from build123d import *

# Parameters (mm, degrees)
EXTRUDE_1_DEPTH = 2000


with BuildPart() as part:
    # Эскиз1 → Вытянуть-Тонкостенный1 (new body)
    with BuildSketch(Plane(origin=(0, 0, 0), x_dir=(0, 0, -1), z_dir=(1, 0, 0))):
        Polygon((-18, -0.2), (0.110849528, -0.2), (5.110849528, 7.8), (57.389150472, 7.8), (62.389150472, -0.2), (115.110849528, -0.2), (120.110849528, 7.8), (172.389150472, 7.8), (177.389150472, -0.2), (230.110849528, -0.2), (235.110849528, 7.8), (287.389150472, 7.8), (292.389150472, -0.2), (345.110849528, -0.2), (350.110849528, 7.8), (402.389150472, 7.8), (407.389150472, -0.2), (460.110849528, -0.2), (465.110849528, 7.8), (517.389150472, 7.8), (522.389150472, -0.2), (575.110849528, -0.2), (580.110849528, 7.8), (632.389150472, 7.8), (637.389150472, -0.2), (690.110849528, -0.2), (695.110849528, 7.8), (747.389150472, 7.8), (752.389150472, -0.2), (805.110849528, -0.2), (810.110849528, 7.8), (862.389150472, 7.8), (867.389150472, -0.2), (920.110849528, -0.2), (925.110849528, 7.8), (977.389150472, 7.8), (982.389150472, -0.2), (1035.110849528, -0.2), (1040.110849528, 7.8), (1092.389150472, 7.8), (1097.389150472, -0.2), (1150.110849528, -0.2), (1155.110849528, 7.8), (1182, 7.8), (1182, 8.2), (1154.889150472, 8.2), (1149.889150472, 0.2), (1097.610849528, 0.2), (1092.610849528, 8.2), (1039.889150472, 8.2), (1034.889150472, 0.2), (982.610849528, 0.2), (977.610849528, 8.2), (924.889150472, 8.2), (919.889150472, 0.2), (867.610849528, 0.2), (862.610849528, 8.2), (809.889150472, 8.2), (804.889150472, 0.2), (752.610849528, 0.2), (747.610849528, 8.2), (694.889150472, 8.2), (689.889150472, 0.2), (637.610849528, 0.2), (632.610849528, 8.2), (579.889150472, 8.2), (574.889150472, 0.2), (522.610849528, 0.2), (517.610849528, 8.2), (464.889150472, 8.2), (459.889150472, 0.2), (407.610849528, 0.2), (402.610849528, 8.2), (349.889150472, 8.2), (344.889150472, 0.2), (292.610849528, 0.2), (287.610849528, 8.2), (234.889150472, 8.2), (229.889150472, 0.2), (177.610849528, 0.2), (172.610849528, 8.2), (119.889150472, 8.2), (114.889150472, 0.2), (62.610849528, 0.2), (57.610849528, 8.2), (4.889150472, 8.2), (-0.110849528, 0.2), (-18, 0.2), align=None)
    extrude(amount=EXTRUDE_1_DEPTH)


solid = part.part
Could you check a few things on this model? Use its own coordinates, in mm. A direction names the side the tool comes from. Round coordinates to 2 decimals unless told otherwise and drop trailing zeros. Write each loop counter-clockwise with the first axis right and the second up, starting at its lowest first coordinate (ties: lowest second). Pieces come first, ordered by that corner, then holes. Notation, with made-up numbers: (1.25, -17) -> (46.25, -17) arc R24 ccw to (46.25, -3) -> close; hole circle Ø10 at (31, 61). An arc over 180 degrees is marked (long way). Use a Markdown table: item, result.
1. If we section it at A-A (z = -495): List the corners of the cut face in (x, y) for me.
Answer key:
| item | result |
|---|---|
| outline | (0, 7.8) -> (2000, 7.8) -> (2000, 8.2) -> (0, 8.2) -> close |
2. Please list where these lines run through material, in increasing order: probe 1 along Y at (x, z) = (1919, -947.5); probe 2 along Y at (x, z) = (1281.5, -1024.5).
Answer key:
| item | result |
|---|---|
| probe 1 | y = 7.8 to 8.2 |
| probe 2 | y = -0.2 to 0.2 |
3. Which directions (+Z, -Z, +X, -X, +Y, -Y) give clear straight access to the entire face, cutting with the end or side of a thin tool? Please do faces 1 (the face through (986, 8.2, -262)), 2 (the face through (986, 7.8, -261)), 3 (the face through (986, 0.2, -664)).
Answer key:
| item | result |
|---|---|
| face 1 | +Z, -Z, +X, -X, +Y |
| face 2 | +X, -X, -Y |
| face 3 | +X, -X, +Y |
4. We'd pull the mould along Z, two halves only. Please class faces 4 (the face through (986, 8.2, -377)), 5 (the face through (986, 0.2, -1124)): +Z half, -Z half, draft (parallel to the pull), parting line (faces both ways), or undercut.
Answer key:
| item | result |
|---|---|
| face 4 | draft |
| face 5 | undercut |
5. If we section it at B-B (y = 1.5): State how many separate pieces and enclosed holes the cut face has, then the cut area to 3 significant figures.
Answer key:
| item | result |
|---|---|
| separate pieces | 21 |
| enclosed holes | 0 |
| area | 19,800 mm^2 |
6. For pin 1 Ø15.5 at (x, z) = (1156, -35) entering from -Y; pin 2 Ø15.5 at (x, z) = (1100.5, -653.5) entering from +Y; pin 3 Ø6 at (x, z) = (933.5, -523.5) entering from +Y, each with a flat end and sliding along its axis, tell me the tip position at first contact or that it passes through.
Answer key:
| item | result |
|---|---|
| pin 1 | stops at y = 7.8 |
| pin 2 | stops at y = 0.2 |
| pin 3 | stops at y = 3.58 |
